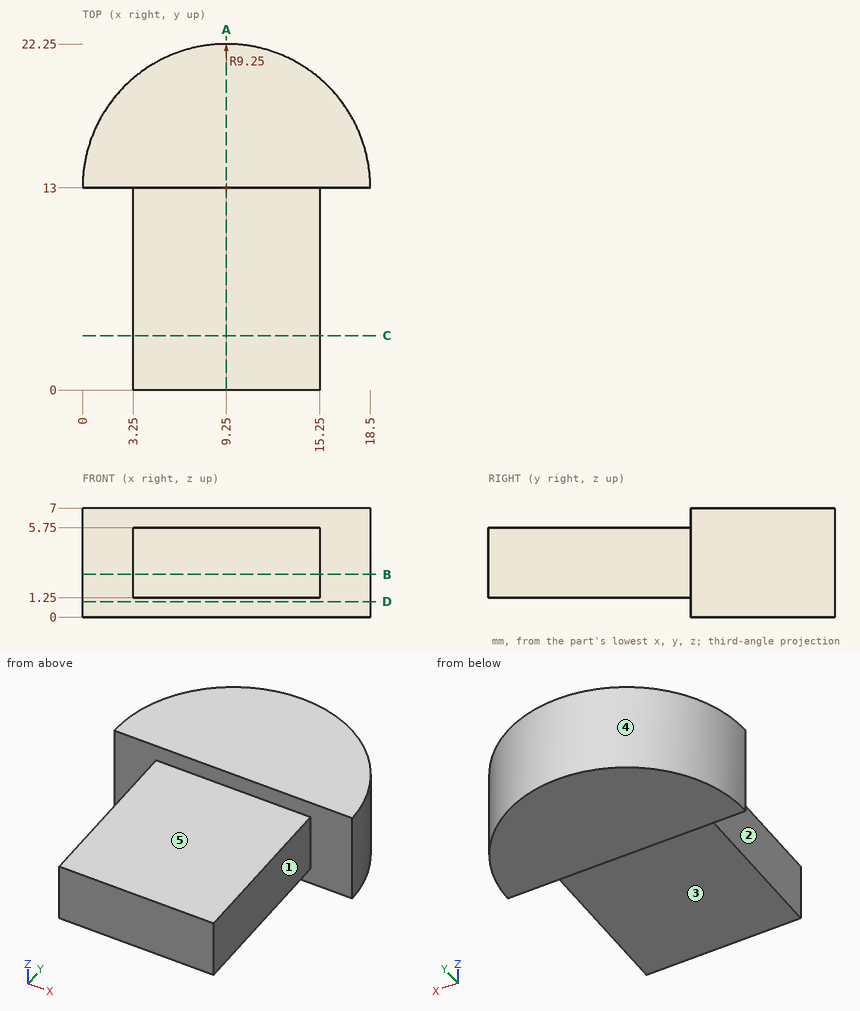
Here's the drawing with two shaded views (mm, measured from the low corner). I have some questions. A direction names the side the tool comes from. Round coordinates to 2 decimals unless told otherwise and drop trailing zeros. Loops run counter-clockwise (first coordinate to the right, second up) from the corner with the lowest first, then second, coordinate; pieces in that order, holes last.
1. For the marked faces 4 and 5, which set-ups out of +Z, -Z, +X, -X, +Y, -Y let a thin tool reach every point of the face, with its end or its side?
Answers:
face 4: +Z, -Z, +Y
face 5: +Z, +X, -X, -Y
2. If I drill on probe 1 along X at (y, z) = (3.5, 5.25); probe 2 along Z at (x, y) = (6.25, 11.75); probe 3 along Y at (x, z) = (9.5, 6.25), over which ranges is the centre line in solid material (lowest first)?
Answers:
probe 1: x = 3.25 to 15.25
probe 2: z = 1.25 to 5.75
probe 3: y = 13 to 22.25
3. Will these pins go through, and if not, where does the flat tip stop? pin 1 (10 mm diameter, centred on x = 8, y = 3.5, fed in from +Z); pin 2 (2 mm diameter, centred on y = 2.5, z = 2.5, fed in from -X); pin 3 (4 mm diameter, centred on y = 18, z = 1.5, fed in from -X).
Answers:
pin 1: stops at z = 5.75
pin 2: stops at x = 3.25
pin 3: stops at x = 0.5
4. Suppose I cut it at B-B, the plane z = 2.75. Please give me the cut outline in (x, y), and give its area (3 significant figures).
Answers:
outline: (0, 13) - (3.25, 13) - (3.25, 0) - (15.25, 0) - (15.25, 13) - (18.5, 13) arc R9.25 ccw to start
area: 290 mm2
5. Suppose I cut it at C-C, the plane y = 3.5. Please give me the cut outline in (x, z), and give its area (3 significant figures).
Answers:
outline: (3.25, 1.25) - (15.25, 1.25) - (15.25, 5.75) - (3.25, 5.75) - close
area: 54.0 mm2
6. Thinking about a two-plate mould opening in X: for the marked faces 1, 2 and 3, which applies, released by +X, released by -X, zero draft, split by the parting line, or undercut?
Answers:
face 1: released by +X
face 2: released by -X
face 3: zero draft
7. Suppose I cut it at D-D, the plane z = 1. Please give me the cut outline in (x, y).
Answers:
outline: (0, 13) - (18.5, 13) arc R9.25 ccw to start
8. Suppose I cut it at A-A, the plane x = 9.25. Please give me the cut outline in (y, z), and give its area (3 significant figures).
Answers:
outline: (0, 1.25) - (13, 1.25) - (13, 0) - (22.25, 0) - (22.25, 7) - (13, 7) - (13, 5.75) - (0, 5.75) - close
area: 123 mm2
